Check sheet for the drawn part. Datum: minimum x, y, z corner. Units: mm. Coordinates: 2 decimals unless noted, no trailing zeros. Write each loop counter-clockwise with the first axis right and the second up, starting at its lowest first coordinate (ties: lowest second). Pieces come first, ordered by that corner, then holes. Notation, with made-up numbers: M 25.5,24 L 78.5,24 A25 cw 78.5,42 Z; hole C 35.25,-22 d6. An arc over 180 degrees is marked long. Answer in a Markdown table with one row per item.
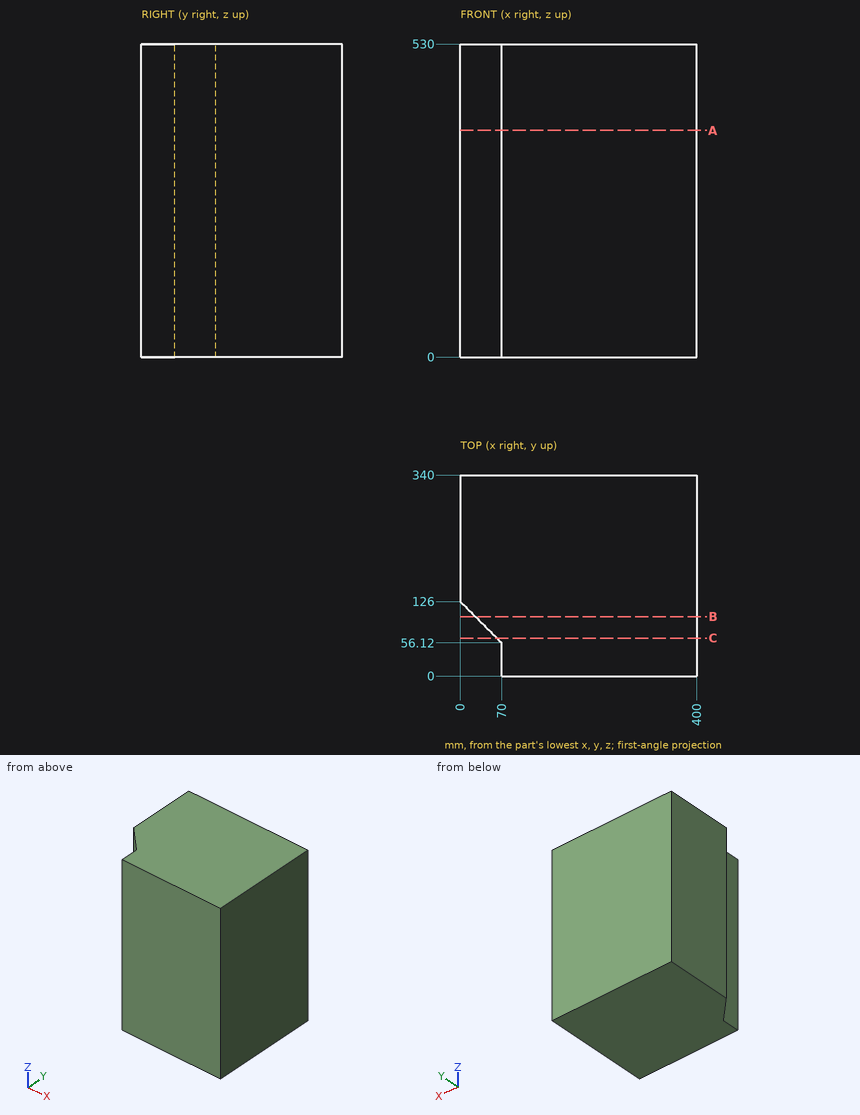
1) Sectioned sample at A-A (z = 384). Record the cut outline in (x, y).
Response values:
| item | result |
|---|---|
| outline | M 0,126 L 70,56.12 L 70,0 L 400,0 L 400,340 L 0,340 Z |
2) Depth check by flat-ended pin: pin 1 (17 mm diameter, centred on y = 36, z = 147, fed in from -X). Enter the tip coordinate at first touch or a pass-through.
Response values:
| item | result |
|---|---|
| pin 1 | stops at x = 70 |
3) Sectioned sample at B-B (y = 100.5). Record the cut outline in (x, z), then the cut area to 3 significant figures.
Response values:
| item | result |
|---|---|
| outline | M 25.54,0 L 400,0 L 400,530 L 25.54,530 Z |
| area | 198,000 mm² |
4) Thickness scan on L1, parallel to Y at x = 44, z = 422.5; L2, parallel to Y at x = 23.5, z = 503. Record the ranges inside material, lowest first. Write a range as [from, to].
Response values:
| item | result |
|---|---|
| L1 | y = [82.08, 340] |
| L2 | y = [102.54, 340] |
5) Sectioned sample at C-C (y = 64). Record the cut outline in (x, z).
Response values:
| item | result |
|---|---|
| outline | M 62.11,0 L 400,0 L 400,530 L 62.11,530 Z |
